Work out the finished part from the listing and answer in its coordinate system (mm). Round coordinates to 2 decimals unless told otherwise and drop trailing zeros. Write each loop counter-clockwise with the first axis right and the second up, starting at its lowest first coordinate (ties: lowest second). Pieces come first, ordered by that corner, then holes. Notation, with made-up numbers: (61, -13) -> (103, -13) arc R17 cw to (103, 5) -> close; hole circle Ø1 at (-17, 30.25). An arc over 180 degrees is marked (long way). One line per item, written item: value.
```python
from build123d import *

# Parameters (mm, degrees)
SKETCH1_R           = 14.2875
SKETCH1_R_2         = 2.6289
BOSS_EXTRUDE1_DEPTH = 6.35


with BuildPart() as part:
    # Sketch1 → Boss-Extrude1 (new body)
    with BuildSketch(Plane(origin=(0, 0, 0), x_dir=(0, 0, -1), z_dir=(1, 0, 0))):
        with BuildLine():
            Line((-12.7, -12.7), (-88.9, -12.7))
            Line((-88.9, -12.7), (-102.396644635, 32.66804481))
            ThreePointArc((-102.396644635, 32.66804481), (-95.394210317, 53.468440807), (-73.450431984, 53.869878795))
            Line((-73.450431984, 53.869878795), (-12.7, 12.7))
            Line((-12.7, 12.7), (25.4, 12.7))
            Line((25.4, 12.7), (81.28, 12.7))
            Line((81.28, 12.7), (88.9, -12.7))
            Line((88.9, -12.7), (25.4, -12.7))
            Line((25.4, -12.7), (-12.7, -12.7))
        make_face()
        with Locations((-84.1375, 38.1)):
            Circle(SKETCH1_R, mode=Mode.SUBTRACT)
        with Locations((-12.7, 0)):
            Circle(SKETCH1_R_2, mode=Mode.SUBTRACT)
        with Locations((12.7, 0)):
            Circle(SKETCH1_R_2, mode=Mode.SUBTRACT)
        with Locations((68.58, 0)):
            Circle(SKETCH1_R_2, mode=Mode.SUBTRACT)
    extrude(amount=BOSS_EXTRUDE1_DEPTH)


solid = part.part
```
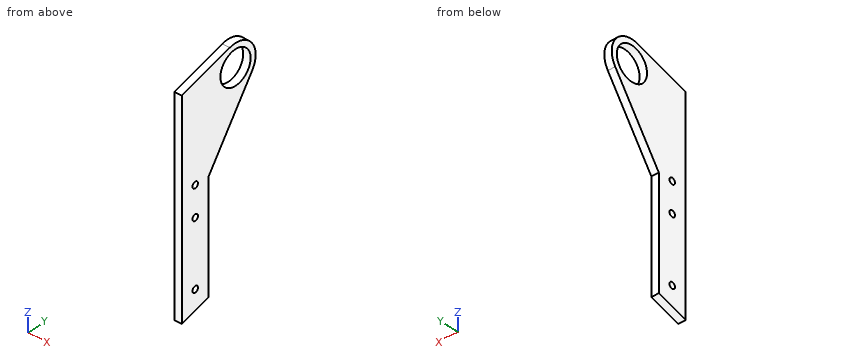
(1) Find section B-B on x = 2. Give the number of separate pieces and of enclosed holes in the cut face, plus the area to 3 significant figures.
Reported:
separate pieces: 1
enclosed holes: 4
area: 6,220 mm2
(2) Flat-ended cylindrical pins translate along their axes: pin 1 Ø12 at (y, z) = (24.5, -39) entering from +X; pin 2 Ø6 at (y, z) = (0, 12.7) entering from -X; pin 3 Ø1 at (x, z) = (5, 62) entering from +Y. Find the tip coordinate at first contact, or state that the pin passes through.
Reported:
pin 1: passes through
pin 2: stops at x = 0
pin 3: stops at y = 46.45
(3) Find section D-D on y = 0. Give the vertices of the cut face in (x, z).
Reported:
outline: (0, -85.09) -> (6.35, -85.09) -> (6.35, -71.21) -> (0, -71.21) -> close; (0, -65.95) -> (6.35, -65.95) -> (6.35, -15.33) -> (0, -15.33) -> close; (0, -10.07) -> (6.35, -10.07) -> (6.35, 10.07) -> (0, 10.07) -> close; (0, 15.33) -> (6.35, 15.33) -> (6.35, 92.68) -> (0, 92.68) -> close
(4) Find section A-A on z = -12.7. Give the vertices of the cut face in (x, y).
Reported:
outline: (0, -12.7) -> (6.35, -12.7) -> (6.35, -2.63) -> (0, -2.63) -> close; (0, 2.63) -> (6.35, 2.63) -> (6.35, 12.7) -> (0, 12.7) -> close
(5) Consider probe 1 along Y at (x, z) = (5, 12.7); probe 2 along Z at (x, y) = (2.75, 39); probe 3 along Y at (x, z) = (5.25, -52). Determine where each line is inside the solid, lowest interval first.
Reported:
probe 1: y = -12.7 to -2.63, 2.63 to 12.7
probe 2: z = 51.51 to 69.88, 98.4 to 103.17
probe 3: y = -12.7 to 12.7
